Input: part model. Units: mm. Frame: model coordinates. A direction names the side the tool comes from. Give positions to 0.01 mm unless a question says otherwise; leave off trailing zeros. Order: outer loops, then holes, each group sorted by start corner. A loop starts at its lowest first (then second) coordinate and runs counter-clockwise, first axis right, second up.
```python
from build123d import *

# Parameters (mm, degrees)
F0_R      = 4
F0_R_2    = 3
F1_DEPTH  = 92.5
F2_R      = 3.5
F2_R_2    = 3
F3_DEPTH  = 1
F4_R      = 4
F4_R_2    = 3
F5_DEPTH  = 1
F6_R      = 3.5
F6_R_2    = 3
F7_DEPTH  = 1
F8_W      = 10.2374576963
F8_H      = 9.6328482032
F8_W_2    = 5.85
F8_H_2    = 5.85
F9_DEPTH  = 1
F10_R     = 4
F10_R_2   = 3
F11_DEPTH = 1


with BuildPart() as f1:
    # F0 (on Front) → F1 (new body)
    with BuildSketch(Plane.XZ):
        Circle(F0_R)
        Circle(F0_R_2, mode=Mode.SUBTRACT)
    extrude(amount=F1_DEPTH)

    # F2 (on face) → F3 (join)
    with BuildSketch(Plane(origin=(0, 0, 0), x_dir=(-1, 0, 0), z_dir=(0, 1, 0))):
        Circle(F2_R)
        Circle(F2_R_2, mode=Mode.SUBTRACT)
    extrude(amount=F3_DEPTH)

    # F4 (on face) → F5 (join)
    with BuildSketch(Plane(origin=(0, 1, 0), x_dir=(-1, 0, 0), z_dir=(0, 1, 0))):
        Circle(F4_R)
        Circle(F4_R_2, mode=Mode.SUBTRACT)
    extrude(amount=F5_DEPTH)

    # F6 (on face) → F7 (join)
    with BuildSketch(Plane(origin=(0, 2, 0), x_dir=(-1, 0, 0), z_dir=(0, 1, 0))):
        Circle(F6_R)
        Circle(F6_R_2, mode=Mode.SUBTRACT)
    extrude(amount=F7_DEPTH)

    # F8 (on face) → F9 (cut)
    with BuildSketch(Plane(origin=(0, 3, 0), x_dir=(-1, 0, 0), z_dir=(0, 1, 0))):
        with Locations((0.2122113947, -0.0024125911)):
            Rectangle(F8_W, F8_H)
        Rectangle(F8_W_2, F8_H_2, mode=Mode.SUBTRACT)
    extrude(amount=-F9_DEPTH, mode=Mode.SUBTRACT)

    # F10 (on face) → F11 (join)
    with BuildSketch(Plane(origin=(0, 3, 0), x_dir=(-1, 0, 0), z_dir=(0, 1, 0))):
        Circle(F10_R)
        Circle(F10_R_2, mode=Mode.SUBTRACT)
    extrude(amount=F11_DEPTH)


solid = f1.part
```
1) Pull-direction query (Y, two-part tool) for faces 3 (the face through (-3.233, 0.493, -1.341)), 4 (the face through (-0.867, -45.602, -3.905)), 5 (the face through (1, -92.5, 3)), 6 (the face through (-0.3, 2, 3.3)); classes: pulls with the +Y half, pulls with the -Y half, needs draft (parallel to the pull), parting line crosses it, or undercut.
2) Cut plane A-A (y = -49). Return the cut outline in (x, z), then the cut area to 3 significant figures.
3) First-contact query: P1, Ø0.8, axis at x = -1, y = 2.5, coming from the -Z side (3 decimals); P2, Ø4, axis at y = -72, z = 0.5, coming from the +X side; P3, Ø0.5, axis at y = 2.5, z = 1.5, coming from the -X side (3 decimals); P4, Ø0.5, axis at y = 2.5, z = -1.5, coming from the +X side (3 decimals). Flat tips, straight axial feed; report the tip coordinate or a pass-through.
4) Reachability of faces 1 (the face through (-0.3, 3, 3.3)), 2 (the face through (-1, 4, 3)) from +Z, -Z, +X, -X, +Y, -Y: full face, straight path, thin tool, end or side. Return the list, or none.
5) Line query: probe 1 along Y at (x, z) = (-2.5, -3); probe 2 along Z at (x, y) = (0, 0.4); probe 3 along Y at (x, z) = (-3, -0.5). Output: solid intervals per line, ascending.
Geometry says:
1. face 3: undercut
1. face 4: needs draft
1. face 5: pulls with the -Y half
1. face 6: undercut
2. outline: circle Ø8 at (0, 0); hole circle Ø6 at (0, 0)
2. area: 22.0 mm2
3. P1: stops at z = -2.925
3. P2: stops at x = 4
3. P3: stops at x = -2.925
3. P4: stops at x = 2.925
4. face 1: none
4. face 2: +Z, -Z, +X, -X, +Y
5. probe 1: y = -92.5 to 0, 1 to 2, 3 to 4
5. probe 2: z = -3.5 to -3, 3 to 3.5
5. probe 3: y = -92.5 to 2, 3 to 4
